```python
from build123d import *

# Parameters (mm, degrees)
SKETCH006_R           = 80
SKETCH006_R_2         = 15.5
PAD002_DEPTH          = 6
SKETCH007_R           = 2.5
POCKET004_DEPTH       = 6
POLARPATTERN002_COUNT = 4
SKETCH008_R           = 5
POCKET005_DEPTH       = 3
POLARPATTERN003_COUNT = 4
SKETCH009_R           = 18
POCKET006_DEPTH       = 3


with BuildPart() as part:
    # Sketch006 → Pad002 (new body)
    with BuildSketch(Plane.XY):
        Circle(SKETCH006_R)
        Circle(SKETCH006_R_2, mode=Mode.SUBTRACT)
    extrude(amount=PAD002_DEPTH)

    # Sketch007 (on Face4 of Pad002) → Pocket004 (cut)
    with BuildSketch(Plane.XY.offset(6)):
        with Locations((42.426407, 42.426407)):
            Circle(SKETCH007_R)
    pocket004 = extrude(amount=-POCKET004_DEPTH, mode=Mode.SUBTRACT)

    # PolarPattern002: Pocket004 ×4 about axis
    polarpattern002_axis = Axis((0, 0, 6), (0, 0, 1))
    for i in range(1, POLARPATTERN002_COUNT):
        add(pocket004.rotate(polarpattern002_axis, i * 360 / POLARPATTERN002_COUNT), mode=Mode.SUBTRACT)

    # Sketch008 (on Face3 of PolarPattern002) → Pocket005 (cut)
    with BuildSketch(Plane.XY.offset(6)):
        with Locations((42.426407, 42.426407)):
            Circle(SKETCH008_R)
    pocket005 = extrude(amount=-POCKET005_DEPTH, mode=Mode.SUBTRACT)

    # PolarPattern003: Pocket005 ×4 about axis
    polarpattern003_axis = Axis((0, 0, 6), (0, 0, 1))
    for i in range(1, POLARPATTERN003_COUNT):
        add(pocket005.rotate(polarpattern003_axis, i * 360 / POLARPATTERN003_COUNT), mode=Mode.SUBTRACT)

    # Sketch009 (on Face3 of PolarPattern003) → Pocket006 (cut)
    with BuildSketch(Plane.XY.offset(6)):
        Circle(SKETCH009_R)
    extrude(amount=-POCKET006_DEPTH, mode=Mode.SUBTRACT)


solid = part.part
```
Verification items for the finished model (mm, model axes). A direction names the side the tool comes from. Round coordinates to 2 decimals unless told otherwise and drop trailing zeros. Loops run counter-clockwise (first coordinate to the right, second up) from the corner with the lowest first, then second, coordinate; pieces in that order, holes last. Notation, with made-up numbers: (-20, 29.25) -> (18, 29.25) arc R18 cw to (18, 34.25) -> close; hole circle Ø8 at (15, 82.25). An arc over 180 degrees is marked (long way). Answer as a JSON object with one key per item and string values.
Q1. Section check D-D (x = 26.5). Record the boundary of the cut face in (y, z), then the cut area to 3 significant figures.
Data:
{"outline": "(-75.48, 0) -> (75.48, 0) -> (75.48, 6) -> (-75.48, 6) -> close", "area": "906 mm2"}
Q2. Section check A-A (y = 0). Record the boundary of the cut face in (x, z), then the cut area to 3 significant figures.
Data:
{"outline": "(-80, 0) -> (-15.5, 0) -> (-15.5, 3) -> (-18, 3) -> (-18, 6) -> (-80, 6) -> close; (15.5, 0) -> (80, 0) -> (80, 6) -> (18, 6) -> (18, 3) -> (15.5, 3) -> close", "area": "759 mm2"}
Q3. Access from +Z, -Z, +X, -X, +Y, -Y to the whole of each face (thin tool, end or side, straight path). Record for faces 1 (the flat face through (5, 15, 3)), 2 (the cylindrical face through (-41.884, -39.986, 1.521)).
Data:
{"face 1": "+Z", "face 2": "+Z, -Z"}
Q4. Go/stop test with flat-tipped pins: P1, Ø3, axis at x = 43.5, y = -43.5, coming from the +Z side; P2, Ø11.5, axis at x = 42.43, y = 42.43, coming from the -Z side; P3, Ø4.5, axis at x = -42.43, y = 42.43, coming from the +Z side; P4, Ø3, axis at x = -27.5, z = 1.5, coming from the +Y side. Record where each tip stops, or that it passes through.
Data:
{"P1": "stops at z = 3", "P2": "stops at z = 0", "P3": "passes through", "P4": "stops at y = 75.66"}
Q5. Draft check along Y on faces 3 (the cylindrical face through (-17.34, -78.1, 2.96)), 4 (the flat face through (-1, 19, 6)), 5 (the flat face through (-40, -41, 3)). Enter one of: pulls with the +Y half, pulls with the -Y half, needs draft (parallel to the pull), parting line crosses it, or undercut.
Data:
{"face 3": "parting line crosses it", "face 4": "needs draft", "face 5": "undercut"}
Q6. Scan lines: line 1 (Y direction, x = 0, z = 1.7); line 2 (Y direction, x = 41, z = 2.6); line 3 (X direction, y = 40, z = 5.2). Record each from-to range of solid material in increasing order. Write a range as from..to.
Data:
{"line 1": "y = -80..-15.5, 15.5..80", "line 2": "y = -68.69..-44.48, -40.37..40.37, 44.48..68.69", "line 3": "x = -69.28..-46.8, -38.05..38.05, 46.8..69.28"}
Q7. Section check C-C (z = 1.65). Record the boundary of the cut face in (x, y), then the cut area to 3 significant figures.
Data:
{"outline": "circle Ø160 at (0, 0); hole circle Ø5 at (-42.43, -42.43); hole circle Ø5 at (-42.43, 42.43); hole circle Ø31 at (0, 0); hole circle Ø5 at (42.43, -42.43); hole circle Ø5 at (42.43, 42.43)", "area": "19,300 mm2"}
